Build history of the part. All positions in model axes, mm. A direction names the side the tool comes from. Give positions to 0.01 mm unless a question says otherwise; leave off trailing zeros. Loops run counter-clockwise (first coordinate to the right, second up) from the corner with the lowest first, then second, coordinate; pieces in that order, holes last. Notation, with made-up numbers: (32.25, 22.5) -> (63.25, 22.5) arc R18 ccw to (63.25, 28.5) -> close; hole circle Ø8 at (17.25, 49.5). An arc over 180 degrees is marked (long way). Answer as a JSON object with one key per item and string values. Group by question number.
Q1. Drop flat-ended pins along their axis: pin 1 (12.5 mm diameter, centred on x = 203.5, z = 17.5, fed in from -Y); pin 2 (5 mm diameter, centred on y = -19, z = 25, fed in from +X); pin 3 (5 mm diameter, centred on y = -19.5, z = 14, fed in from -X). Give the stop position or say it passes through.
Q2. Band-saw the part on C-C, the plane y = -18.5. Write the cut outline in (x, z), plus the area to 3 significant figures.
Q3. Wall check: probe 1 along Z at (x, y) = (0, -16.25); probe 2 along X at (y, z) = (-3, 23); probe 3 along X at (y, z) = (-18.5, 27). Give the ranges that are in metal, low to high. Write a range as from..to.
Q4. Two-plate mould, pull along X, no slides. Class faces 1 (the cylindrical face through (-2.38, -12.68, 6.76)), 2 (the flat face through (-187.5, -20, 17)), 3 (the flat face through (212.5, -7, 17)), 4 (the flat face through (-3, 0, 6)): pulls with the +X half, pulls with the -X half, needs draft (parallel to the pull), parting line crosses it, or undercut.
Q5. Band-saw the part on A-A, the plane z = 17.5. Write the cut outline in (x, y).
Q6. Band-saw the part on B-B, the plane x = 0. Write the cut outline in (y, z).
Q7. Tool access for faces 5 (the flat face through (-200, -15, 18)), 6 (the flat face through (200, -15, 18)), 7 (the flat face through (-3, -25, 6)): list every direction of +Z, -Z, +X, -X, +Y, -Y with a clear straight run to the whole face (end or side of a thin tool).
from build123d import *

# Parameters (mm, degrees)
F0_W     = 425
F0_H     = 35
F1_DEPTH = 15
F2_W     = 375
F2_H     = 35
F3_DEPTH = 10
F5_D     = 22


with BuildPart() as f1:
    # F0 (on Front) → F1 (new body)
    with BuildSketch(Plane.XZ):
        with Locations((0, 17.5)):
            Rectangle(F0_W, F0_H)
    extrude(amount=F1_DEPTH)

    # F2 (on face) → F3 (join)
    with BuildSketch(Plane.XZ.offset(15)):
        with Locations((0, 17.5)):
            Rectangle(F2_W, F2_H)
    extrude(amount=F3_DEPTH)

    # F5 (through all)
    with Locations(Plane(origin=(0, 0, 0), x_dir=(-1, 0, 0), z_dir=(0, 1, 0))):
        with Locations((0, 17.5)):
            Hole(F5_D / 2)


solid = f1.part
Worked answers:
{
 "1": {"pin 1": "y = -15", "pin 2": "x = 187.5", "pin 3": "x = -187.5"},
 "2": {"outline": "(-187.5, 0) -> (187.5, 0) -> (187.5, 35) -> (-187.5, 35) -> close; hole circle Ø22 at (0, 17.5)", "area": "12,700 mm2"},
 "3": {"probe 1": "0..6.5, 28.5..35", "probe 2": "-212.5..-9.53, 9.53..212.5", "probe 3": "-187.5..-5.55, 5.55..187.5"},
 "4": {"face 1": "undercut", "face 2": "pulls with the -X half", "face 3": "pulls with the +X half", "face 4": "needs draft"},
 "5": {"outline": "(-212.5, -15) -> (-187.5, -15) -> (-187.5, -25) -> (-11, -25) -> (-11, 0) -> (-212.5, 0) -> close; (11, -25) -> (187.5, -25) -> (187.5, -15) -> (212.5, -15) -> (212.5, 0) -> (11, 0) -> close"},
 "6": {"outline": "(-25, 0) -> (0, 0) -> (0, 6.5) -> (-25, 6.5) -> close; (-25, 28.5) -> (0, 28.5) -> (0, 35) -> (-25, 35) -> close"},
 "7": {"face 5": "+Z, -Z, -X, -Y", "face 6": "+Z, -Z, +X, -Y", "face 7": "+Z, -Z, +X, -X, -Y"}
}
